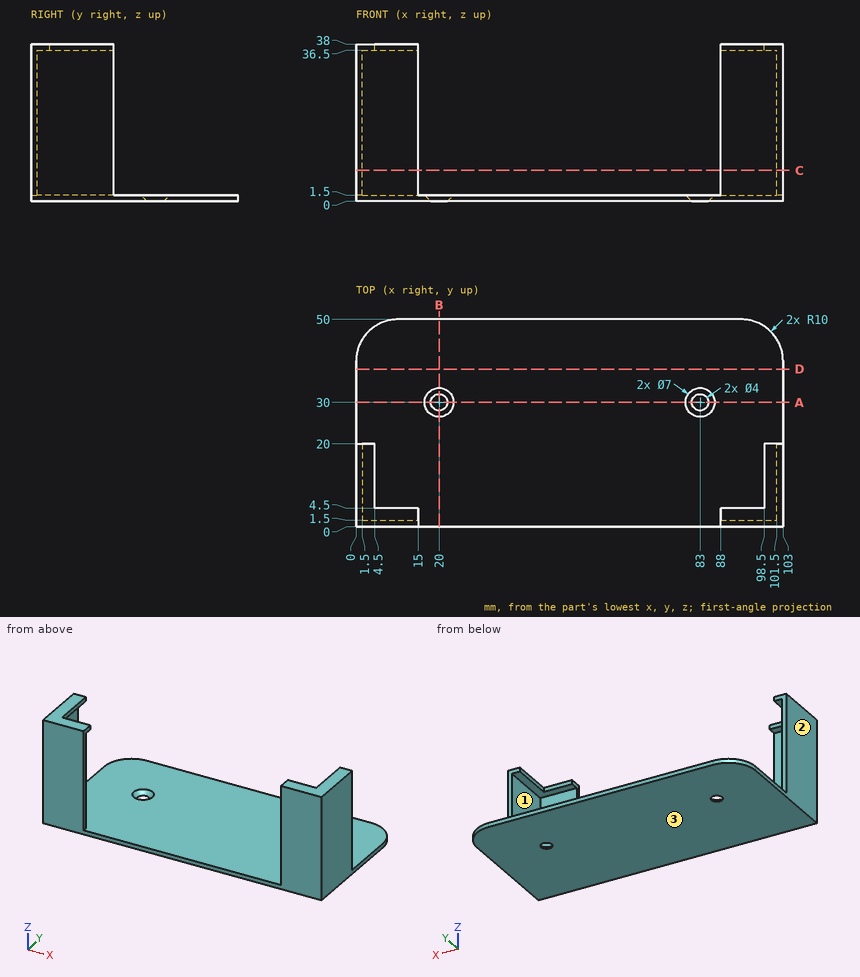
Geometry check sheet. Reference: drawing and pictorial views, mm from the part's lowest x, y, z. Give positions to 0.01 mm unless a question says otherwise; leave off trailing zeros. Write each loop counter-clockwise with the first axis right and the second up, starting at its lowest first coordinate (ties: lowest second). Pieces come first, ordered by that corner, then holes. Notation, with made-up numbers: M -13.5,6.5 L -2.5,6.5 A30 ccw -2.5,41.5 Z; hole C 9.5,2.25 d8. An arc over 180 degrees is marked long. Put each result on its own line as item: value. Start each with the question number.
1. Scan lines: line 1 along X through (y, z) = (17.5, 25.5); line 2 along Z through (x, y) = (71, 39). Record each from-to range of solid material in increasing order. Write a range as [from, to].
2. Draft check along X on the marked faces 1, 2 and 3. Enter one of: +X half, -X half, draft (parallel to the pull), parting line (faces both ways), or undercut.
3. Section check D-D (y = 38). Record the cut outline in (x, z), and give its area (4 significant figures).
4. Section check A-A (y = 30). Record the cut outline in (x, z).
5. Go/stop test with flat-tipped pins: pin 1 Ø4 at (x, y) = (84.5, 43.5) entering from +Z; pin 2 Ø3.5 at (x, z) = (1, 28) entering from +Y; pin 3 Ø11 at (x, z) = (8, 11.5) entering from +Y. Record where each tip stops, or that it passes through.
6. Section check B-B (x = 20). Record the cut outline in (y, z).
7. Section check C-C (z = 7.5). Record the cut outline in (x, y).
Answer list:
1. line 1: [0, 1.5], [101.5, 103]
1. line 2: [0, 1.5]
2. face 1: undercut
2. face 2: -X half
2. face 3: draft
3. outline: M 0,0 L 103,0 L 103,1.5 L 0,1.5 Z
3. area: 154.5 mm2
4. outline: M 0,0 L 18,0 L 16.5,1.5 L 0,1.5 Z; M 22,0 L 81,0 L 79.5,1.5 L 23.5,1.5 Z; M 85,0 L 103,0 L 103,1.5 L 86.5,1.5 Z
5. pin 1: z = 1.5
5. pin 2: y = 20
5. pin 3: y = 1.5
6. outline: M 0,0 L 28,0 L 26.5,1.5 L 0,1.5 Z; M 32,0 L 50,0 L 50,1.5 L 33.5,1.5 Z
7. outline: M 0,0 L 15,0 L 15,1.5 L 1.5,1.5 L 1.5,20 L 0,20 Z; M 88,0 L 103,0 L 103,20 L 101.5,20 L 101.5,1.5 L 88,1.5 Z
